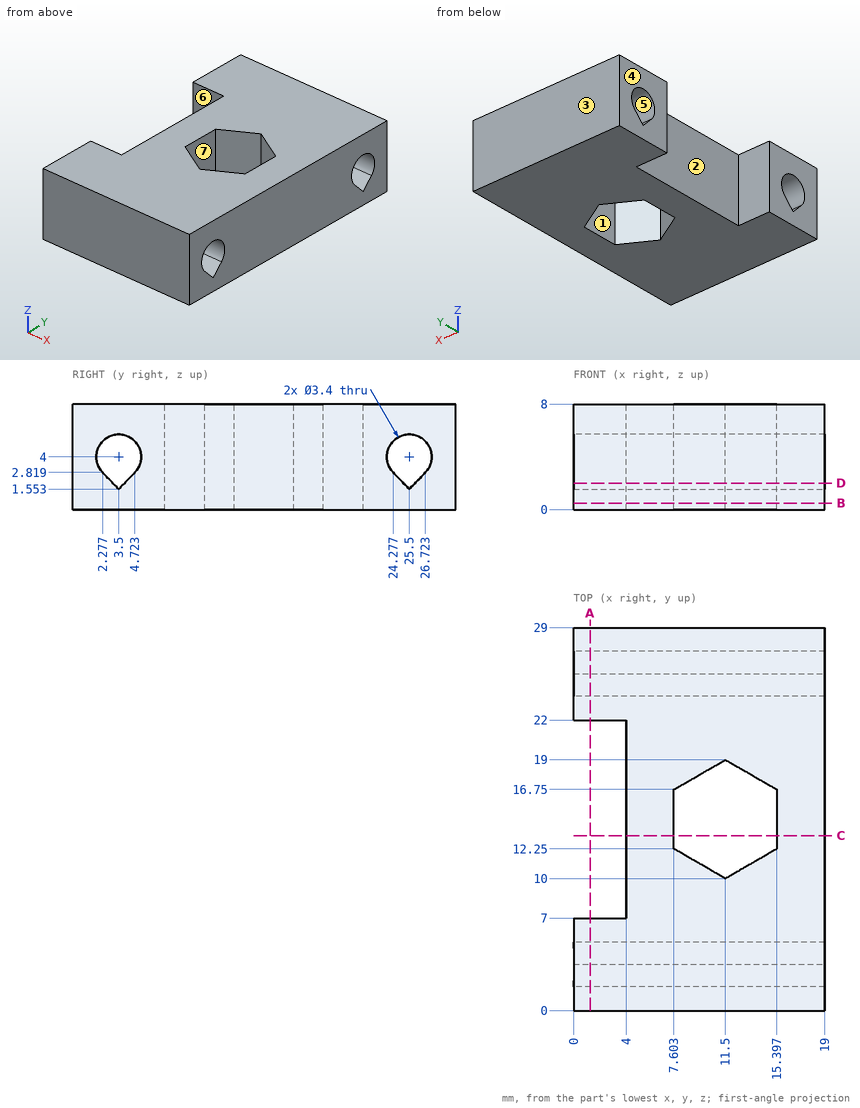
Can you work these out from the drawing? Everything is in mm from the part's minimum corner. A direction names the side the tool comes from. Give positions to 0.01 mm unless a question says otherwise; leave off trailing zeros. Write each loop counter-clockwise with the first axis right and the second up, starting at its lowest first coordinate (ties: lowest second). Pieces come first, ordered by that corner, then holes. Notation, with made-up numbers: M -22.75,14.5 L -5.75,14.5 A16 cw -5.75,30.5 Z; hole C -15.5,-24 d6. An arc over 180 degrees is marked long. Answer in a Markdown table with one row per item. Add a question column.
Item 1: Imagine slicing it at B-B, the plane z = 0.5. Write out the boundary of the cut face in (x, y).
Item 2: For pin 1 Ø1 at (y, z) = (11.5, 1) entering from -X; pin 2 Ø2 at (y, z) = (25.5, 4) entering from -X, each with a flat end and sliding along its axis, tell me the tip position at first contact or that it passes through.
Item 3: We'd pull the mould along Y, two halves only. Please class the marked faces 1, 2, 3 and 4: released by +Y, released by -Y, zero draft, split by the parting line, or undercut.
Item 4: Imagine slicing it at C-C, the plane y = 13.25. Write out the boundary of the cut face in (x, z).
Item 5: Imagine slicing it at A-A, the plane x = 1.25. Write out the boundary of the cut face in (y, z).
Item 6: Please list where these lines run through material, in increasing order: L1, parallel to Y at x = 1.25, z = 7.25; L2, parallel to X at y = 12.5, z = 4.25; L3, parallel to Y at x = 8, z = 4.
Item 7: On a 3-axis mill with a long thin cutter (end or side, diameter ignored), from which of +Z, -Z, +X, -X, +Y, -Y can I reach the whole of each face in a straight line? I mean the marked faces 5, 6 and 7. Say none if no direction works.
Item 8: Imagine slicing it at D-D, the plane z = 2. Write out the boundary of the cut face in (x, y).
Evaluation:
| question | item | result |
|---|---|---|
| 1 | outline | M 0,0 L 19,0 L 19,29 L 0,29 L 0,22 L 4,22 L 4,7 L 0,7 Z; hole M 7.6,12.25 L 11.5,10 L 15.4,12.25 L 15.4,16.75 L 11.5,19 L 7.6,16.75 Z |
| 2 | pin 1 | stops at x = 4 |
| 2 | pin 2 | passes through |
| 3 | face 1 | undercut |
| 3 | face 2 | undercut |
| 3 | face 3 | released by +Y |
| 3 | face 4 | zero draft |
| 4 | outline | M 4,0 L 7.6,0 L 7.6,8 L 4,8 Z; M 15.4,0 L 19,0 L 19,8 L 15.4,8 Z |
| 5 | outline | M 0,0 L 7,0 L 7,8 L 0,8 Z; M 22,0 L 29,0 L 29,8 L 22,8 Z; hole M 2.28,2.82 L 3.5,1.55 L 4.72,2.82 A1.7 ccw long Z; hole M 24.28,2.82 L 25.5,1.55 L 26.72,2.82 A1.7 ccw long Z |
| 6 | L1 | y = 0 to 7, 22 to 29 |
| 6 | L2 | x = 4 to 7.6, 15.4 to 19 |
| 6 | L3 | y = 0 to 1.8, 5.2 to 12.02, 16.98 to 23.8, 27.2 to 29 |
| 7 | face 5 | +X, -X |
| 7 | face 6 | +Z, -Z, -X |
| 7 | face 7 | +Z, -Z |
| 8 | outline | M 0,0 L 19,0 L 19,3.07 L 0,3.07 Z; M 0,3.93 L 19,3.93 L 19,25.07 L 0,25.07 L 0,22 L 4,22 L 4,7 L 0,7 Z; M 0,25.93 L 19,25.93 L 19,29 L 0,29 Z; hole M 7.6,12.25 L 11.5,10 L 15.4,12.25 L 15.4,16.75 L 11.5,19 L 7.6,16.75 Z |
